Check sheet for the modelled part. Datum: model origin and axes. Units: mm. Face numbers are marked on the shaded views. A direction names the side the tool comes from. Round coordinates to 2 decimals unless told otherwise and drop trailing zeros. Order: outer loops, then holes, each group sorted by start corner. A loop starts at its lowest first (then second) coordinate and runs counter-clockwise, first axis right, second up.
Q1. Mould release check, pull along X, two halves, no side actions. Record for the marked faces 3, 4, 5 and 6: +X half, -X half, draft (parallel to the pull), parting line (faces both ways), or undercut.
Q2. Cross-section at A-A on y = 0. Record the cut outline in (x, z), then the cut area to 3 significant figures.
Q3. Depth check by flat-ended pin: P1, Ø0.5, axis at y = -4.5, z = 0.5, coming from the -X side; P2, Ø2, axis at x = -13, z = 2.5, coming from the -Y side; P3, Ø13, axis at x = -30, y = 5.5, coming from the -Z side. Enter the tip coordinate at first touch or a pass-through.
Q4. Cross-section at D-D on z = 2.85. Record the cut outline in (x, y), then the cut area to 3 significant figures.
Q5. Set-up check for the marked faces 1 and 2: record each of +Z, -Z, +X, -X, +Y, -Y from which the full face is reachable in a straight line by a thin tool's end or side.
Q6. Cross-section at C-C on x = -28. Record the cut outline in (y, z), then the cut area to 3 significant figures.
Q7. Cross-section at B-B on z = 0.6. Record the cut outline in (x, y).
Q8. Scan lines: probe 1 along Y at (x, z) = (-28, 2.7); probe 2 along Y at (x, z) = (-5.39, 2.9); probe 3 along X at (y, z) = (-1.5, 1.1). Record each from-to range of solid material in increasing order.
from build123d import *

# Parameters (mm, degrees)
EXTRUDE1_DEPTH                  = 4
SKETCH2_W                       = 12
SKETCH2_H                       = 1
EXTRUDE2_DEPTH                  = 25
F_4_CLEARANCE_HOLE1_D           = 3.2639
F_4_CLEARANCE_HOLE1_DEPTH       = 8.382
F_4_CLEARANCE_HOLE1_TIP         = 0.980574487
F_8_32_TAPPED_HOLE1_D           = 3.4544
F_8_32_TAPPED_HOLE1_DEPTH       = 10.7188
F_8_32_TAPPED_HOLE1_CBORE_D     = 4.1656
F_8_32_TAPPED_HOLE1_CBORE_DEPTH = 8.3312
F_8_32_TAPPED_HOLE1_TIP         = 1.037806461
FILLET1_R                       = 2.54
CHAMFER1_SIZE                   = 0.2


with BuildPart() as part:
    # Sketch1 → Extrude1 (new body)
    with BuildSketch(Plane.XY):
        Polygon((0, 0), (-17.137776081, 12), (-34, 12), (-34, 0), (-34, -12), (-17.137776081, -12), align=None)
    extrude(amount=EXTRUDE1_DEPTH)

    # Sketch2 → Extrude2 (cut, through all)
    with BuildSketch(Plane(origin=(0, 12, 0), x_dir=(1, 0, 0), z_dir=(0, 1, 0))):
        with Locations((-28, -0.5)):
            Rectangle(SKETCH2_W, SKETCH2_H)
    extrude(amount=-EXTRUDE2_DEPTH, mode=Mode.SUBTRACT)

    # #4 Clearance Hole1
    with Locations(Plane(origin=(-28, 5, 4), x_dir=(1, 0, 0), z_dir=(0, 0, 1))):
        with Locations((0, 0), (0, -10)):
            Hole(F_4_CLEARANCE_HOLE1_D / 2, depth=F_4_CLEARANCE_HOLE1_DEPTH)
            with Locations((0, 0, -(F_4_CLEARANCE_HOLE1_DEPTH + F_4_CLEARANCE_HOLE1_TIP / 2))):  # 118° drill point
                Cone(0, F_4_CLEARANCE_HOLE1_D / 2, F_4_CLEARANCE_HOLE1_TIP, mode=Mode.SUBTRACT)

    # #8-32 Tapped Hole1
    with Locations(Plane(origin=(-5.39, 0, 4), x_dir=(1, 0, 0), z_dir=(0, 0, 1))):
        with Locations((0, 0)):
            CounterBoreHole(F_8_32_TAPPED_HOLE1_D / 2, F_8_32_TAPPED_HOLE1_CBORE_D / 2, F_8_32_TAPPED_HOLE1_CBORE_DEPTH, depth=F_8_32_TAPPED_HOLE1_DEPTH)
            with Locations((0, 0, -(F_8_32_TAPPED_HOLE1_DEPTH + F_8_32_TAPPED_HOLE1_TIP / 2))):  # 118° drill point
                Cone(0, F_8_32_TAPPED_HOLE1_D / 2, F_8_32_TAPPED_HOLE1_TIP, mode=Mode.SUBTRACT)

    # Fillet1
    fillet1_edges = [part.edges().sort_by_distance(p)[0] for p in [
        (-17.137776081, -12, 2),
        (-34, -12, 2.5),
        (-34, 12, 2.5),
        (-17.137776081, 12, 2),
        (0, 0, 2),
    ]]
    fillet(fillet1_edges, radius=FILLET1_R)

    # Chamfer1
    chamfer1_edges = [part.edges().sort_by_distance(p)[0] for p in [
        (-19.969317502, -12, 0),
        (-26.36805, -5, 4),
        (-26.36805, 5, 4),
        (-7.4728, 0, 4),
        (-24.699317502, -12, 4),
        (-34, 0, 4),
        (-9.726610784, -6.810646192, 4),
        (-9.726610784, 6.810646192, 4),
        (-24.699317502, 12, 4),
        (-33.256051224, 11.256051224, 4),
        (-17.174842274, 11.882441055, 4),
        (-1.888354861, 0, 4),
        (-17.174842274, -11.882441055, 4),
        (-33.256051224, -11.256051224, 4),
        (-9.726610784, -6.810646192, 0),
        (-19.969317502, 12, 0),
        (-9.726610784, 6.810646192, 0),
        (-17.174842274, 11.882441055, 0),
        (-1.888354861, 0, 0),
        (-17.174842274, -11.882441055, 0),
    ]]
    chamfer(chamfer1_edges, length=CHAMFER1_SIZE)


solid = part.part
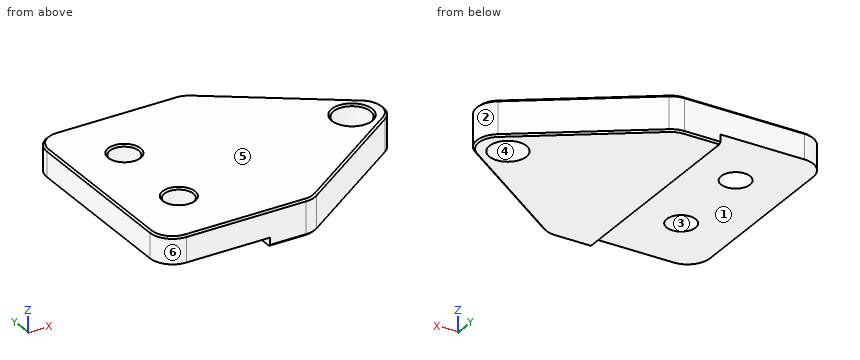
Results found:
1. face 3: undercut
1. face 4: undercut
1. face 5: draft
1. face 6: -X half
2. outline: (-34, 1) - (-22, 1) - (-22, 0) - (-7.47, 0) - (-7.47, 3.8) - (-7.67, 4) - (-33.8, 4) - (-34, 3.8) - close; (-3.31, 0) - (-2.09, 0) - (-1.89, 0.2) - (-1.89, 3.8) - (-2.09, 4) - (-3.11, 4) - (-3.31, 3.8) - close
2. area: 99.7 mm2
3. P1: stops at x = -22
3. P2: stops at y = -9.8
3. P3: stops at z = 1
4. outline: (-34, -9.46) arc R2.54 ccw to (-31.46, -12) - (-17.94, -12) arc R2.54 ccw to (-16.48, -11.54) - (-2.97, -2.08) arc R2.54 ccw to (-2.97, 2.08) - (-16.48, 11.54) arc R2.54 ccw to (-17.94, 12) - (-31.46, 12) arc R2.54 ccw to (-34, 9.46) - close; hole circle Ø3.26 at (-28, -5); hole circle Ø3.26 at (-28, 5); hole circle Ø4.17 at (-5.39, 0)
4. area: 574 mm2
5. face 1: -Z, -X, +Y, -Y
5. face 2: +Z, -Z, +X
6. outline: (-12, 1) - (-6.63, 1) - (-6.63, 3.8) - (-6.83, 4) - (-11.8, 4) - (-12, 3.8) - close; (-3.37, 1) - (3.37, 1) - (3.37, 3.8) - (3.17, 4) - (-3.17, 4) - (-3.37, 3.8) - close; (6.63, 1) - (12, 1) - (12, 3.8) - (11.8, 4) - (6.83, 4) - (6.63, 3.8) - close
6. area: 52.3 mm2
7. outline: (-22, -12) - (-17.94, -12) arc R2.54 ccw to (-16.48, -11.54) - (-2.97, -2.08) arc R2.54 ccw to (-2.97, 2.08) - (-16.48, 11.54) arc R2.54 ccw to (-17.94, 12) - (-22, 12) - close; hole circle Ø4.17 at (-5.39, 0)
8. probe 1: y = -12 to -6.63, -3.37 to 3.37, 6.63 to 12
8. probe 2: y = -3.77 to -2.08, 2.08 to 3.77
8. probe 3: x = -34 to -6.84, -3.94 to -2.38
